Here's the drawing with two shaded views (mm, measured from the low corner). I have some questions. A direction names the side the tool comes from. Round coordinates to 2 decimals unless told otherwise and drop trailing zeros. Order: outer loops, then holes, each group sorted by start corner. A loop starts at its lowest first (then second) coordinate and runs counter-clockwise, first axis right, second up.
Q1. Will these pins go through, and if not, where does the flat tip stop? P1, Ø16, axis at y = 10.5, z = 40, coming from the +X side; P2, Ø10, axis at x = 13, y = 12.5, coming from the +Z side; P3, Ø15, axis at y = 16, z = 46, coming from the -X side.
Q2. We'd pull the mould along X, two halves only. Please class the marked faces 4, 5 and 6: pulls with the +X half, pulls with the -X half, needs draft (parallel to the pull), parting line crosses it, or undercut.
Q3. If we section it at A-A (z = 46): Please give me the cut outline in (x, y), plus the area to 3 significant figures.
Q4. If we section it at B-B (y = 16): Please give me the cut outline in (x, z), plus the area to 3 significant figures.
Q5. If we section it at D-D (y = 8): Please give me the cut outline in (x, z).
Q6. If we section it at C-C (z = 36.5): Please give me the cut outline in (x, y), plus the area to 3 significant figures.
Q7. If I drill on line 1 (X direction, y = 6, z = 27.5); line 2 (X direction, y = 21, z = 10); line 3 (Z direction, x = 26.25, y = 16), over which ranges is the centre line in solid material (lowest first)?
Q8. For the marked faces 1, 2 and 3, which set-ups out of +Z, -Z, +X, -X, +Y, -Y let a thin tool reach every point of the face, with its end or its side?
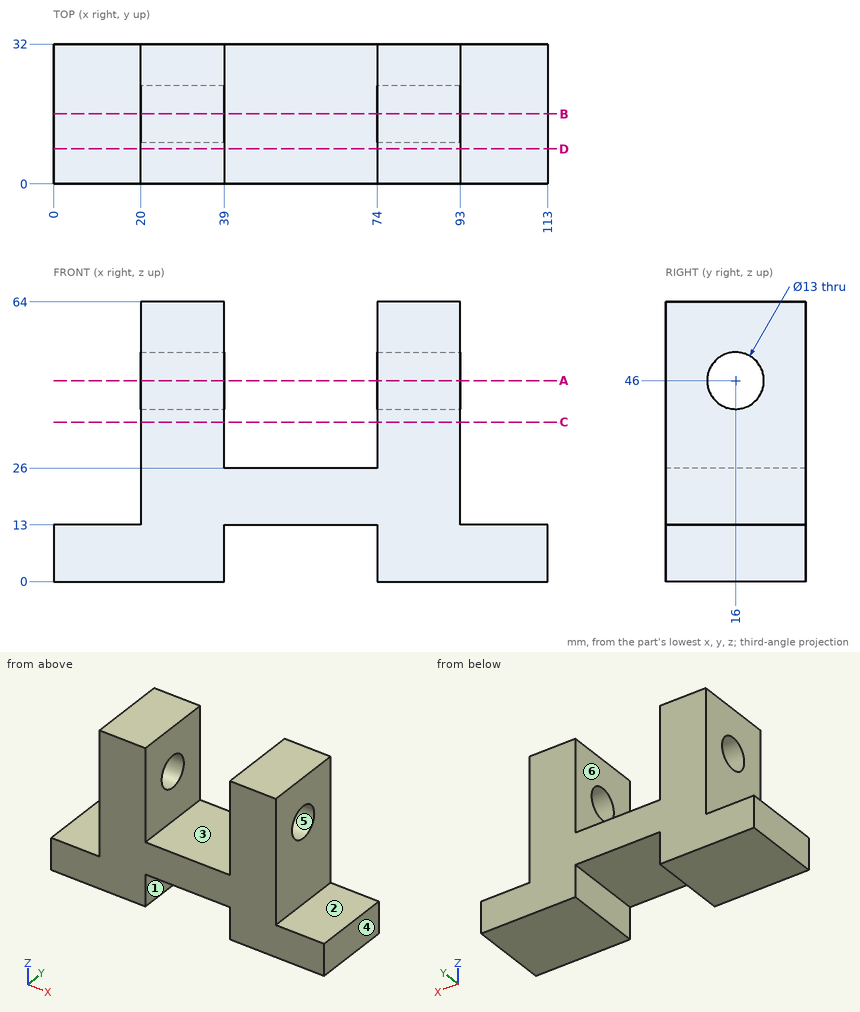
Solution:
1. P1: stops at x = 93
1. P2: stops at z = 13
1. P3: stops at x = 20
2. face 4: pulls with the +X half
2. face 5: needs draft
2. face 6: undercut
3. outline: (20, 0) - (39, 0) - (39, 9.5) - (20, 9.5) - close; (20, 22.5) - (39, 22.5) - (39, 32) - (20, 32) - close; (74, 0) - (93, 0) - (93, 9.5) - (74, 9.5) - close; (74, 22.5) - (93, 22.5) - (93, 32) - (74, 32) - close
3. area: 722 mm2
4. outline: (0, 0) - (39, 0) - (39, 13) - (74, 13) - (74, 0) - (113, 0) - (113, 13) - (93, 13) - (93, 39.5) - (74, 39.5) - (74, 26) - (39, 26) - (39, 39.5) - (20, 39.5) - (20, 13) - (0, 13) - close; (20, 52.5) - (39, 52.5) - (39, 64) - (20, 64) - close; (74, 52.5) - (93, 52.5) - (93, 64) - (74, 64) - close
4. area: 2,910 mm2
5. outline: (0, 0) - (39, 0) - (39, 13) - (74, 13) - (74, 0) - (113, 0) - (113, 13) - (93, 13) - (93, 64) - (74, 64) - (74, 26) - (39, 26) - (39, 64) - (20, 64) - (20, 13) - (0, 13) - close
6. outline: (20, 0) - (39, 0) - (39, 32) - (20, 32) - close; (74, 0) - (93, 0) - (93, 32) - (74, 32) - close
6. area: 1,220 mm2
7. line 1: x = 20 to 39, 74 to 93
7. line 2: x = 0 to 39, 74 to 113
7. line 3: z = 0 to 39.5, 52.5 to 64
8. face 1: -Z, +Y, -Y
8. face 2: +Z, +X, +Y, -Y
8. face 3: +Z, +Y, -Y
